The model under review builds one solid part; all positions refer to its coordinate system, in mm. Face numbers are marked on the shaded views. A direction names the side the tool comes from. Round coordinates to 2 decimals unless told otherwise and drop trailing zeros. Order: outer loops, then holes, each group sorted by start corner. A loop starts at its lowest first (then second) coordinate and runs counter-clockwise, first axis right, second up.
1) Clearance check with flat-ended pins moving along their axes: P1, Ø3, axis at x = -2, y = -3.5, coming from the +Z side; P2, Ø1.5, axis at x = 8.5, z = 15.5, coming from the -Y side; P3, Ø4, axis at x = -8.5, z = 21, coming from the +Y side; P4, Ø3, axis at x = -12, y = 5, coming from the -Z side. State where each tip first meets the part, or that it passes through.
2) Mouldability with a two-part tool opening along X and no side actions: class the marked faces 1, 2 and 3 as pulls with the +X half, pulls with the -X half, needs draft (parallel to the pull), parting line crosses it, or undercut.
3) Consider section B-B (x = -11). Give the boundary of the cut face in (y, z), then the cut area to 3 significant figures.
4) Consider section A-A (y = 4.5). Give the boundary of the cut face in (x, z).
5) To check wall thickness, follow L1, parallel to Y at x = -10, z = -20; L2, parallel to X at y = 7.5, z = 26; L3, parallel to Y at x = -10.75, z = 25. State the ranges of each line that lie inside material, in increasing order.
6) Consider section C-C (y = -5.5). Give the boundary of the cut face in (x, z).
7) Consider section D-D (z = -24). Give the boundary of the cut face in (x, y), then the cut area to 3 significant figures.
8) Machinability: for the marked faces 4 and 5, which of the approach directions +Z, -Z, +X, -X, +Y, -Y give a long, thin tool a straight path to every point of the face, cutting with its end or side? Answer none if there is none.
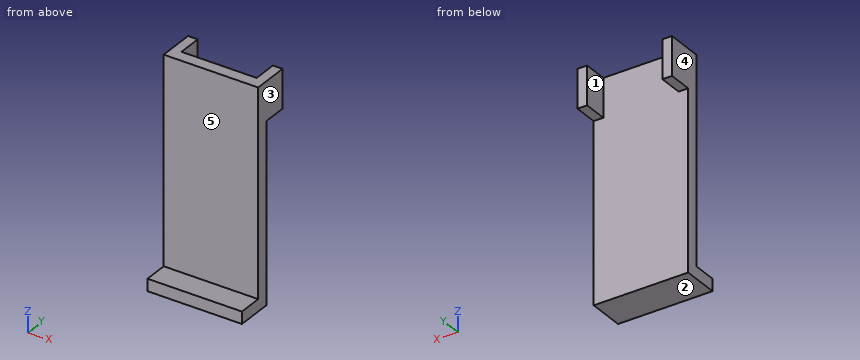
from build123d import *

# Parameters (mm, degrees)
SKETCH2_W           = 24.892
SKETCH2_H           = 57.15
BOSS_EXTRUDE1_DEPTH = 3.175
SKETCH3_W           = 2.54
SKETCH3_H           = 10.16
BOSS_EXTRUDE2_DEPTH = 6.35
SKETCH4_W           = 24.892
SKETCH4_H           = 3.175
BOSS_EXTRUDE3_DEPTH = 6.35
SCALE1_SCALE        = 1.02


with BuildPart() as part:
    # Sketch2 → Boss-Extrude1 (new body)
    with BuildSketch(Plane(origin=(0, 0, 0), x_dir=(1, 0, 0), z_dir=(0, 1, 0))):
        Rectangle(SKETCH2_W, SKETCH2_H)
    extrude(amount=BOSS_EXTRUDE1_DEPTH)

    # Sketch3 → Boss-Extrude2 (add)
    with BuildSketch(Plane(origin=(0, 3.175, 0), x_dir=(1, 0, 0), z_dir=(0, 1, 0))):
        with Locations((11.176, -23.495)):
            Rectangle(SKETCH3_W, SKETCH3_H)
        with Locations((-11.176, -23.495)):
            Rectangle(SKETCH3_W, SKETCH3_H)
    extrude(amount=BOSS_EXTRUDE2_DEPTH)

    # Sketch4 → Boss-Extrude3 (add)
    with BuildSketch(Plane.XZ):
        with Locations((0, -26.9875)):
            Rectangle(SKETCH4_W, SKETCH4_H)
    extrude(amount=BOSS_EXTRUDE3_DEPTH)


with BuildPart() as part_1:
    # Scale1: scaled about (0, 1.432399425, -1.093002874)
    add(part.part.scale(SCALE1_SCALE).moved(Location((0, -0.028647989, 0.021860057))))


solid = part_1.part
Answer below:
1. P1: stops at z = -25.89
1. P2: stops at y = -0.03
1. P3: stops at y = 9.69
1. P4: stops at z = 18.81
2. face 1: undercut
2. face 2: needs draft
2. face 3: pulls with the +X half
3. outline: (-6.51, -29.12) - (3.21, -29.12) - (3.21, 18.81) - (9.69, 18.81) - (9.69, 29.17) - (-0.03, 29.17) - (-0.03, -25.89) - (-6.51, -25.89) - close
3. area: 277 mm2
4. outline: (-12.69, 18.81) - (-10.1, 18.81) - (-10.1, 29.17) - (-12.69, 29.17) - close; (10.1, 18.81) - (12.69, 18.81) - (12.69, 29.17) - (10.1, 29.17) - close
5. L1: y = -0.03 to 3.21
5. L2: x = -12.69 to -10.1, 10.1 to 12.69
5. L3: y = -0.03 to 9.69
6. outline: (-12.69, -29.12) - (12.69, -29.12) - (12.69, -25.89) - (-12.69, -25.89) - close
7. outline: (-12.69, -0.03) - (12.69, -0.03) - (12.69, 3.21) - (-12.69, 3.21) - close
7. area: 82.2 mm2
8. face 4: +Z, -Z, -X, +Y, -Y
8. face 5: +Z, +X, -X, -Y
